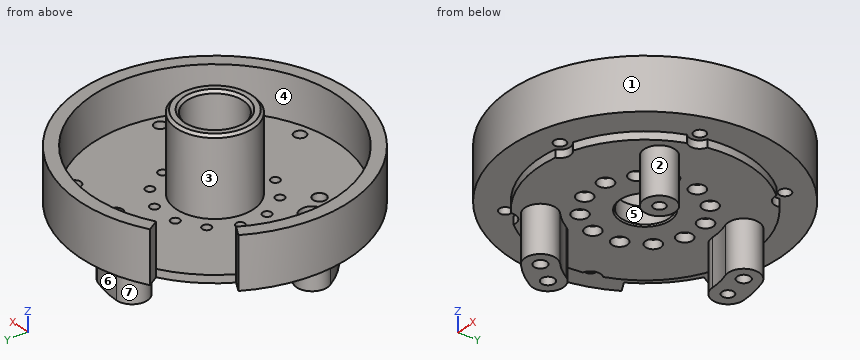
from build123d import *

# Parameters (mm, degrees)
SKETCH_1_R                   = 41
EXTRUDE_1_DEPTH              = 6
SKETCH_2_R                   = 15
EXTRUDE_2_DEPTH              = 30
SKETCH_3_R                   = 9.275
CUT_EXTRUDE_2_DEPTH          = 7
SKETCH_6_R                   = 11
CUT_EXTRUDE_3_DEPTH          = 65.830548355
CHAMFER_1_SIZE               = 0.5
SKETCH_7_R                   = 6
EXTRUDE_3_DEPTH              = 18
PATTERN_CIRCULAR_1_COUNT     = 3
SKETCH_8_R                   = 4.5
CUT_EXTRUDE_4_DEPTH          = 17
PATTERN_CIRCULAR_2_COUNT     = 3
SKETCH_9_R                   = 2.25
CUT_EXTRUDE_5_DEPTH          = 75.639131828
PATTERN_CIRCULAR_3_COUNT     = 3
F_5_0MM_1_D                  = 5
F_5_0MM_1_CSINK_D            = 5.05
F_5_0MM_1_CSINK_ANGLE        = 90
F_5_0MM_2_D                  = 5
F_5_0MM_2_CSINK_D            = 5.05
F_5_0MM_2_CSINK_ANGLE        = 90
EXTRUDE_5_DEPTH              = 18
F_5_0MM_3_AT_2_COUNT         = 2
F_5_0MM_3_AT_2_PITCH         = 62.596471695
EXTRUDE_6_DEPTH              = 17
EXTRUDE_6_DEPTH_BACK         = 3
SKETCH_20_R                  = 52.5
SKETCH_20_R_2                = 47.55
CUT_EXTRUDE_6_DEPTH          = 85.814503477
EXTRUDE_START                = -3
SKETCH_25_R                  = 47.55
SKETCH_25_R_2                = 41
EXTRUDE_7_DEPTH              = 3
HOLE_WIZARD_M3_1_D           = 3.4
HOLE_WIZARD_M3_1_CBORE_D     = 6
HOLE_WIZARD_M3_1_CBORE_DEPTH = 3.4
PATTERN_CIRCULAR_4_COUNT     = 12
CHAMFER_2_SIZE               = 1
SKETCH_30_R                  = 2.25
CUT_EXTRUDE_9_DEPTH          = 81.07808689
PATTERN_CIRCULAR_16_COUNT    = 6
SKETCH_31_R                  = 4
CUT_EXTRUDE_10_DEPTH         = 3
PATTERN_CIRCULAR_17_COUNT    = 6


with BuildPart() as part:
    # Sketch 1 → Extrude 1 (new body)
    with BuildSketch(Plane.XY):
        Circle(SKETCH_1_R)
    extrude(amount=EXTRUDE_1_DEPTH)

    # Sketch 2 → Extrude 2 (add)
    with BuildSketch(Plane.XY.offset(6)):
        Circle(SKETCH_2_R)
    extrude(amount=EXTRUDE_2_DEPTH)

    # Sketch 3 → Cut-Extrude 2 (cut)
    with BuildSketch(Plane(origin=(0, 0, 0), x_dir=(-1, 0, 0), z_dir=(0, 0, -1))):
        Circle(SKETCH_3_R)
    extrude(amount=-CUT_EXTRUDE_2_DEPTH, mode=Mode.SUBTRACT)

    # Sketch 6 → Cut-Extrude 3 (cut, through all)
    with BuildSketch(Plane(origin=(0, 0, 7), x_dir=(-1, 0, 0), z_dir=(0, 0, -1))):
        Circle(SKETCH_6_R)
    extrude(amount=-CUT_EXTRUDE_3_DEPTH, mode=Mode.SUBTRACT)

    # Chamfer 1
    chamfer_1_edges = [part.edges().sort_by_distance(p)[0] for p in [
        (9.275, 0, 0),
    ]]
    chamfer(chamfer_1_edges, length=CHAMFER_1_SIZE)

    # Sketch 7 → Extrude 3 (add)
    with BuildSketch(Plane(origin=(0, 0, 0), x_dir=(-1, 0, 0), z_dir=(0, 0, -1))):
        with Locations(Location((0, 32, 0), (0, 0, 180))):
            Circle(SKETCH_7_R)
    extrude_3 = extrude(amount=EXTRUDE_3_DEPTH)

    # Pattern Circular 1: Extrude 3 ×3 about axis
    pattern_circular_1_axis = Axis((0, 0, 0), (0, 0, 1))
    for i in range(1, PATTERN_CIRCULAR_1_COUNT):
        add(extrude_3.rotate(pattern_circular_1_axis, i * 360 / PATTERN_CIRCULAR_1_COUNT))

    # Sketch 8 → Cut-Extrude 4 (cut)
    with BuildSketch(Plane.XY.offset(6)):
        with Locations((0, 32)):
            Circle(SKETCH_8_R)
    cut_extrude_4 = extrude(amount=-CUT_EXTRUDE_4_DEPTH, mode=Mode.SUBTRACT)

    # Pattern Circular 2: Cut-Extrude 4 ×3 about axis
    pattern_circular_2_axis = Axis((0, 0, 0), (0, 0, 1))
    for i in range(1, PATTERN_CIRCULAR_2_COUNT):
        add(cut_extrude_4.rotate(pattern_circular_2_axis, i * 360 / PATTERN_CIRCULAR_2_COUNT), mode=Mode.SUBTRACT)

    # Sketch 9 → Cut-Extrude 5 (cut, through all)
    with BuildSketch(Plane.XY.offset(-11)):
        with Locations((0, 32)):
            Circle(SKETCH_9_R)
    cut_extrude_5 = extrude(amount=-CUT_EXTRUDE_5_DEPTH, mode=Mode.SUBTRACT)

    # Pattern Circular 3: Cut-Extrude 5 ×3 about axis
    pattern_circular_3_axis = Axis((0, 0, 0), (0, 0, 1))
    for i in range(1, PATTERN_CIRCULAR_3_COUNT):
        add(cut_extrude_5.rotate(pattern_circular_3_axis, i * 360 / PATTERN_CIRCULAR_3_COUNT), mode=Mode.SUBTRACT)

    # 5.0mm _1 (through all)
    with Locations(Plane.XY.offset(6)):
        with Locations((-21.421060687, -23.772634646), (-27.712813081, -15.99999984)):
            CounterSinkHole(F_5_0MM_1_D / 2, F_5_0MM_1_CSINK_D / 2, counter_sink_angle=F_5_0MM_1_CSINK_ANGLE)

    # 5.0mm _2 (through all)
    with Locations(Plane.XY.offset(6)):
        with Locations((9.877175378, 30.437499903)):
            CounterSinkHole(F_5_0MM_2_D / 2, F_5_0MM_2_CSINK_D / 2, counter_sink_angle=F_5_0MM_2_CSINK_ANGLE)

    # Sketch 18 → Extrude 5 (add)
    with BuildSketch(Plane(origin=(0, 0, 0), x_dir=(-1, 0, 0), z_dir=(0, 0, -1))):
        with BuildLine():
            ThreePointArc((-11.729145803, 36.144531262), (-15.584206737, 28.585529478), (-8.025205013, 24.730468729))
            ThreePointArc((-8.025205013, 24.730468729), (-4.062500003, 25.680656004), (0, 26))
            ThreePointArc((0, 26), (-6, 32), (0, 38))
            ThreePointArc((0, 38), (-5.937500012, 37.533266511), (-11.729145803, 36.144531262))
        make_face()
        with BuildLine():
            ThreePointArc((17.404611815, -19.315265657), (16.963691699, -27.789083518), (25.437509581, -28.230003658))
            ThreePointArc((25.437509581, -28.230003658), (29.536012358, -23.90865898), (32.908965344, -19))
            ThreePointArc((32.908965344, -19), (24.712812921, -21.196152423), (22.516660498, -13))
            ThreePointArc((22.516660498, -13), (20.208850557, -16.358556141), (17.404611815, -19.315265657))
        make_face()
    extrude(amount=EXTRUDE_5_DEPTH)

    # Sketch 19 → 5.0mm _3 (revolve, cut)
    with BuildSketch(Plane(origin=(9.877175378, 30.437499903, 0), x_dir=(0, -1, 0), z_dir=(1, 0, 0))):
        Polygon((0, 0), (0, 18), (2.5, 18), (2.5, 0.025), (2.525, 0), align=None)
    f_5_0mm_3 = revolve(axis=Axis((9.877175378, 30.437499903, 6.35), (0, 0, -1)), mode=Mode.SUBTRACT)

    # 5.0mm _3 at 2: 5.0mm _3 ×2
    with Locations(*[Vector(-0.5000000034830118, -0.8660254017735209, 0) * (i * F_5_0MM_3_AT_2_PITCH) for i in range(1, F_5_0MM_3_AT_2_COUNT)]):
        add(f_5_0mm_3, mode=Mode.SUBTRACT)



with BuildPart() as body_2:
    # Sketch 20 → Extrude 6 (new, two sides: drawn at the far end of the back side and taken through both)
    with BuildSketch(Plane.XY.offset(6).offset(-EXTRUDE_6_DEPTH_BACK)):
        Circle(SKETCH_20_R)
        Circle(SKETCH_20_R_2, mode=Mode.SUBTRACT)
    extrude(amount=EXTRUDE_6_DEPTH + EXTRUDE_6_DEPTH_BACK)

    # Sketch 23 → Cut-Extrude 6 (cut, through all)
    with BuildSketch(Plane.XY.offset(23)):
        with BuildLine():
            Line((-41.163149036, 23.803311985), (-45.448271806, 26.281259289))
            ThreePointArc((-45.448271806, 26.281259289), (-37.097569065, 37.148625405), (-26.218728298, 45.484374091))
            Line((-26.218728298, 45.484374091), (-23.746676773, 41.195847391))
            ThreePointArc((-23.746676773, 41.195847391), (-33.599798267, 33.646040724), (-41.163149036, 23.803311985))
        make_face()
    extrude(amount=-CUT_EXTRUDE_6_DEPTH, mode=Mode.SUBTRACT)


with BuildPart() as part_1:
    add(part.part)

    add(body_2.part)  # Extrude 7 merges body 2
    # Sketch 25 → Extrude 7 (add)
    with BuildSketch(Plane.XY.offset(6).offset(EXTRUDE_START)):
        Circle(SKETCH_25_R)
        Circle(SKETCH_25_R_2, mode=Mode.SUBTRACT)
    extrude(amount=EXTRUDE_7_DEPTH)

    # Hole Wizard M3 _1 (through all)
    with Locations(Plane(origin=(0, 0, 0), x_dir=(-1, 0, 0), z_dir=(0, 0, -1))):
        with Locations((5.189664299, -19.314952355)):
            hole_wizard_m3_1 = CounterBoreHole(HOLE_WIZARD_M3_1_D / 2, HOLE_WIZARD_M3_1_CBORE_D / 2, HOLE_WIZARD_M3_1_CBORE_DEPTH)

    # Pattern Circular 4: Hole Wizard M3 _1 ×12 about axis
    pattern_circular_4_axis = Axis((0, 0, 0), (0, 0, 1))
    for i in range(1, PATTERN_CIRCULAR_4_COUNT):
        add(hole_wizard_m3_1.rotate(pattern_circular_4_axis, i * 360 / PATTERN_CIRCULAR_4_COUNT), mode=Mode.SUBTRACT)

    # Chamfer 2
    chamfer_2_edges = [part_1.edges().sort_by_distance(p)[0] for p in [
        (11, 0, 36),
        (-15, 0, 36),
    ]]
    chamfer(chamfer_2_edges, length=CHAMFER_2_SIZE)

    # Sketch 30 → Cut-Extrude 9 (cut, through all)
    with BuildSketch(Plane.XY.offset(6)):
        with Locations((-41.527147563, 11.157778242)):
            Circle(SKETCH_30_R)
    cut_extrude_9 = extrude(amount=-CUT_EXTRUDE_9_DEPTH, mode=Mode.SUBTRACT)

    # Pattern Circular 16: Cut-Extrude 9 ×6 about axis
    pattern_circular_16_axis = Axis((0, 0, 0), (0, 0, 1))
    for i in range(1, PATTERN_CIRCULAR_16_COUNT):
        add(cut_extrude_9.rotate(pattern_circular_16_axis, i * 360 / PATTERN_CIRCULAR_16_COUNT), mode=Mode.SUBTRACT)

    # Sketch 31 → Cut-Extrude 10 (cut)
    with BuildSketch(Plane(origin=(0, 0, 3), x_dir=(-1, 0, 0), z_dir=(0, 0, -1))):
        with Locations((41.527147563, 11.157778242)):
            Circle(SKETCH_31_R)
    cut_extrude_10 = extrude(amount=CUT_EXTRUDE_10_DEPTH, mode=Mode.SUBTRACT)

    # Pattern Circular 17: Cut-Extrude 10 ×6 about axis
    pattern_circular_17_axis = Axis((0, 0, 0), (0, 0, 1))
    for i in range(1, PATTERN_CIRCULAR_17_COUNT):
        add(cut_extrude_10.rotate(pattern_circular_17_axis, i * 360 / PATTERN_CIRCULAR_17_COUNT), mode=Mode.SUBTRACT)


solid = part_1.part
Source: CAD feature listing. Evaluate the final solid. Frame: model axes, mm. Face numbers are marked on the shaded views. A direction names the side the tool comes from. Round coordinates to 2 decimals unless told otherwise and drop trailing zeros. Loops run counter-clockwise (first coordinate to the right, second up) from the corner with the lowest first, then second, coordinate; pieces in that order, holes last. Notation, with made-up numbers: M 79.5,-23 L 102.5,-23 A20 cw 102.5,-7 Z; hole C 48.25,-20.5 d6. An arc over 180 degrees is marked long. Answer as CSV lines item,"result".
Q1. Cut plane B-B (z = -2). Return the cut outline in (x, y).
Verdict:
outline,"M -32.91,-19 A38 ccw -25.44,-28.23 A6 ccw -17.4,-19.32 A26 cw -22.52,-13 A6 ccw Z; M 0,26 A26 cw 8.03,24.73 A6 ccw 11.73,36.14 A38 ccw 0,38 A6 ccw Z; C 27.71,-16 d12; hole C -27.71,-16 d9; hole C -21.42,-23.77 d5; hole C 0,32 d9; hole C 9.88,30.44 d5; hole C 27.71,-16 d9"
Q2. Cut plane C-C (z = 30). Return the cut outline in (x, y).
Verdict:
outline,"C 0,0 d30; hole C 0,0 d22"
Q3. Line query: line 1 along X through (y, z) = (-4, 5); line 2 along Y through (x, z) = (0, -16); line 3 along X through (y, z) = (-4.5, 13). Output: solid intervals per line, ascending.
Verdict:
line 1,"x = -52.35 to -20.56, -18.08 to -8.37, 8.37 to 18.1, 20.53 to 52.35"
line 2,"y = 26 to 29.75, 34.25 to 38"
line 3,"x = -52.31 to -47.34, -14.31 to -10.04, 10.04 to 14.31, 47.34 to 52.31"
Q4. Pull-direction query (X, two-part tool) for the marked faces 4, 5, 6 and 7; classes: +X half, -X half, draft (parallel to the pull), parting line (faces both ways), or undercut.
Verdict:
face 4,"undercut"
face 5,"undercut"
face 6,"+X half"
face 7,"-X half"
Q5. Contact query for flat-ended pins moving along their axis: pin 1 (5 mm diameter, centred on x = -19.32, y = -5.16, fed in from -Z); pin 2 (4 mm diameter, centred on x = 27.5, z = 21, fed in from +Y); pin 3 (1.5 mm diameter, centred on x = -31.5, z = 18.5, fed in from +Y); pin 4 (4 mm diameter, centred on x = -20, y = -24.5, fed in from -Z). Output: stop coordinate, or through.
Verdict:
pin 1,"stops at z = 3.4"
pin 2,"stops at y = 45.89"
pin 3,"stops at y = -34.94"
pin 4,"stops at z = -18"
Q6. Reachability of the marked faces 1, 2 and 3 from +Z, -Z, +X, -X, +Y, -Y: full face, straight path, thin tool, end or side. Return the list, or none.
Verdict:
face 1,"+Z, -Z"
face 2,"-Z"
face 3,"+Z"
